Read the model definition and answer for the solid it produces. Units are mm, in the model's axes. Face numbers are marked on the shaded views. A direction names the side the tool comes from. Coordinates: 2 decimals unless noted, no trailing zeros. Loops run counter-clockwise (first coordinate to the right, second up) from the corner with the lowest first, then second, coordinate; pieces in that order, holes last. Notation, with made-up numbers: (54.25, -23) - (111.25, -23) arc R37 ccw to (111.25, 16) - close; hole circle Ø5 at (40, 83). An arc over 180 degrees is marked (long way). Use CSV: the item, a comma, the result in double quotes.
```python
from build123d import *

# Parameters (mm, degrees)
F0_R     = 15
F1_DEPTH = 2
F2_R     = 3.75
F3_DEPTH = 10
F4_R     = 0.99999


# Not quite as in the source:
# - a fillet or chamfer is up to 0.001 mm smaller than in the source, because OpenCascade refuses the exact size


with BuildPart() as f1:
    # F0 (on Top) → F1 (new body)
    with BuildSketch(Plane.XY):
        Circle(F0_R)
    extrude(amount=F1_DEPTH)

    # F2 (on face) → F3 (join)
    with BuildSketch(Plane.XY.offset(2)):
        Circle(F2_R)
    extrude(amount=F3_DEPTH)

    # F4 (radius 1 in the source; OpenCascade refuses exactly that, so slightly less here)
    f4_edges = [f1.edges().sort_by_distance(p)[0] for p in [
        (-3.75, 0, 12),
        (15, 0, 1),
        (-15, 0, 0),
        (-15, 0, 2),
    ]]
    fillet(f4_edges, radius=F4_R)


solid = f1.part
```
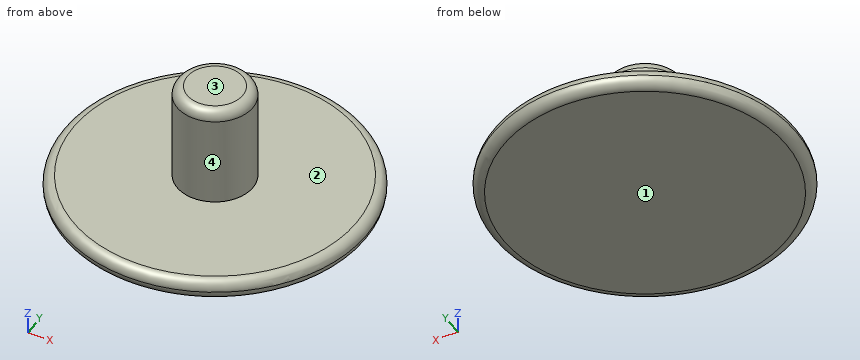
Q1. For a pull along Y with two mould halves and no side action, classify the marked faces 3 and 4 as +Y half, -Y half, draft (parallel to the pull), parting line (faces both ways), or undercut.
Reported:
face 3,"draft"
face 4,"parting line"
Q2. A tool of negligible diameter and unlimited length cuts with its end or side. For the marked faces 1 and 2, from which of +Z, -Z, +X, -X, +Y, -Y can it reach the whole face along a straight path? Write none if from no direction.
Reported:
face 1,"-Z, +X, -X, +Y, -Y"
face 2,"+Z"
Q3. Given P1, Ø6, axis at x = 8, z = 7, coming from the +Y side; P2, Ø1, axis at y = 3.5, z = 8, coming from the +X side; P3, Ø4, axis at x = -2.5, y = 11, coming from the +Z side; P4, Ø2, axis at x = 2.5, z = 10, coming from the +Y side, each flat-ended and moving along its own axis, determine where each tip first touches the part or whether it passes through.
Reported:
P1,"passes through"
P2,"stops at x = 2.25"
P3,"stops at z = 2"
P4,"stops at y = 3.44"
Q4. Find the intervals of material crossed by probe 1 along Z at (x, y) = (-3, 12); probe 2 along X at (y, z) = (-12, 1.5); probe 3 along Y at (x, z) = (-12, 1.25), in increasing order. Write a range as [from, to].
Reported:
probe 1,"z = [0, 2]"
probe 2,"x = [-8.77, 8.77]"
probe 3,"y = [-8.95, 8.95]"
Q5. The part is cut by section C-C on z = 5. Determine the outline of the cut face in (x, y), and give its area (3 significant figures).
Reported:
outline,"circle Ø7.5 at (0, 0)"
area,"44.2 mm²"
